from build123d import *

# Parameters (mm, degrees)
F0_W           = 38
F0_H           = 29
F1_DEPTH       = 480
F2_DEPTH       = 74
F3_DEPTH       = 38
F4_R           = 5
F7_D           = 12
F8_D           = 5
F8_CSINK_D     = 10
F8_CSINK_ANGLE = 90


with BuildPart() as f1:
    # F0 (on Right) → F1 (new body)
    with BuildSketch(Plane.YZ):
        with Locations((10, -14.5)):
            Rectangle(F0_W, F0_H)
        with Locations((10, 14.5)):
            Rectangle(F0_W, F0_H)
        Polygon((-9, 0), (-9, 29), (-29, 29), (-29, -29), (-9, -29), align=None)
    extrude(amount=-F1_DEPTH)

    # F0 (on Right) → F2 (cut)
    with BuildSketch(Plane.YZ):
        Polygon((-9, 0), (-9, 29), (-29, 29), (-29, -29), (-9, -29), align=None)
    extrude(amount=-F2_DEPTH, mode=Mode.SUBTRACT)

    # F0 (on Right) → F3 (cut)
    with BuildSketch(Plane.YZ):
        with Locations((10, -14.5)):
            Rectangle(F0_W, F0_H)
    extrude(amount=-F3_DEPTH, mode=Mode.SUBTRACT)

    # F4
    f4_edges = [f1.edges().sort_by_distance(p)[0] for p in [
        (0, 29, 14.5),
    ]]
    fillet(f4_edges, radius=F4_R)

    # F7 (through all)
    with Locations(Plane(origin=(0, 0, 0), x_dir=(1, 0, 0), z_dir=(0, 0, -1))):
        with Locations((-19, -10)):
            Hole(F7_D / 2)

    # F8 (through all)
    with Locations(Plane(origin=(0, 29, 0), x_dir=(-1, 0, 0), z_dir=(0, 1, 0))):
        with Locations((19, 14.5), (56, 14.5), (56, -14.5)):
            CounterSinkHole(F8_D / 2, F8_CSINK_D / 2, counter_sink_angle=F8_CSINK_ANGLE)

    # F9: F1 across face


with BuildPart() as f1_1:
    add(f1.part)
    add(f1.part.mirror(Plane(origin=(-480, 0, 0), x_dir=(0, 1, 0), z_dir=(-1, 0, 0))))


solid = f1_1.part
Geometry: final body of the model. Coordinates: model frame, mm. A direction names the side the tool comes from. Give positions to 0.01 mm unless a question says otherwise; leave off trailing zeros. Return JSON: item names as keys, results as strings. Group by question number.
1) Set-up query: faces 1 (the flat face through (-38, 10, -14)), 2 (the flat face through (-45, -9, 6)), 3 (the flat face through (-886, -19, 0)). Return all of +Z, -Z, +X, -X, +Y, -Y with unobstructed straight access to the full face (end or side cutting, diameter ignored); none if empty.
2) Mould query, pull axis Z, two halves, no side actions, for faces 4 (the flat face through (-487, 0, 29)), 5 (the flat face through (-915, -9, 6)), 6 (the flat face through (-486, 0, -29)). Classes: released by +Z, released by -Z, zero draft, split by the parting line, or undercut.
3) First-contact query: P1, Ø4.5, axis at x = -19, z = 14.5, coming from the -Y side; P2, Ø23, axis at y = 7.5, z = -13, coming from the -X side; P3, Ø19, axis at x = -941, y = 10, coming from the -Z side; P4, Ø6, axis at x = -56, z = 14.5, coming from the -Y side. Flat tips, straight axial feed; report the tip coordinate or a pass-through.
4) Line query: line 1 (X direction, y = -2.75, z = 14.5); line 2 (X direction, y = 4, z = -14); line 3 (X direction, y = 23, z = 14). Output: solid intervals per line, ascending.
Filled in:
{
 "1": {"face 1": "-Z, +X, +Y, -Y", "face 2": "+Z, -Z, +X, -Y", "face 3": "+Z, -Z, -X, -Y"},
 "2": {"face 4": "released by +Z", "face 5": "zero draft", "face 6": "released by -Z"},
 "3": {"P1": "passes through", "P2": "stops at x = -922", "P3": "stops at z = 0", "P4": "stops at y = -9"},
 "4": {"line 1": "x = -960 to -943.5, -938.5 to -906.5, -901.5 to -58.5, -53.5 to -21.5, -16.5 to 0", "line 2": "x = -922 to -906.45, -901.55 to -58.45, -53.55 to -38", "line 3": "x = -960 to -943.45, -938.55 to -906.45, -901.55 to -58.45, -53.55 to -21.45, -16.55 to 0"}
}
